Check sheet for the drawn part. Datum: minimum x, y, z corner. Units: mm. Coordinates: 2 decimals unless noted, no trailing zeros. Loops run counter-clockwise (first coordinate to the right, second up) from the corner with the lowest first, then second, coordinate; pieces in that order, holes last. Notation, with made-up numbers: M -12.5,33 L -6.5,33 A9 ccw -6.5,39 Z; hole C 64,5.25 d8. An arc over 180 degrees is marked long. Use CSV: the item, a comma, the result in double quotes. Start each with the question number.
(1) Section check B-B on x = 1.1. Record the cut outline in (y, z), and give its area (3 significant figures).
(2) Section check A-A on z = 0.5. Record the cut outline in (x, y), and give its area (3 significant figures).
(3) Scan lines: line 1 (Y direction, x = 0.75, z = 7.5); line 2 (X direction, y = 0.6, z = 3.5); line 3 (Y direction, x = 1.25, z = 7). Record each from-to range of solid material in increasing order.
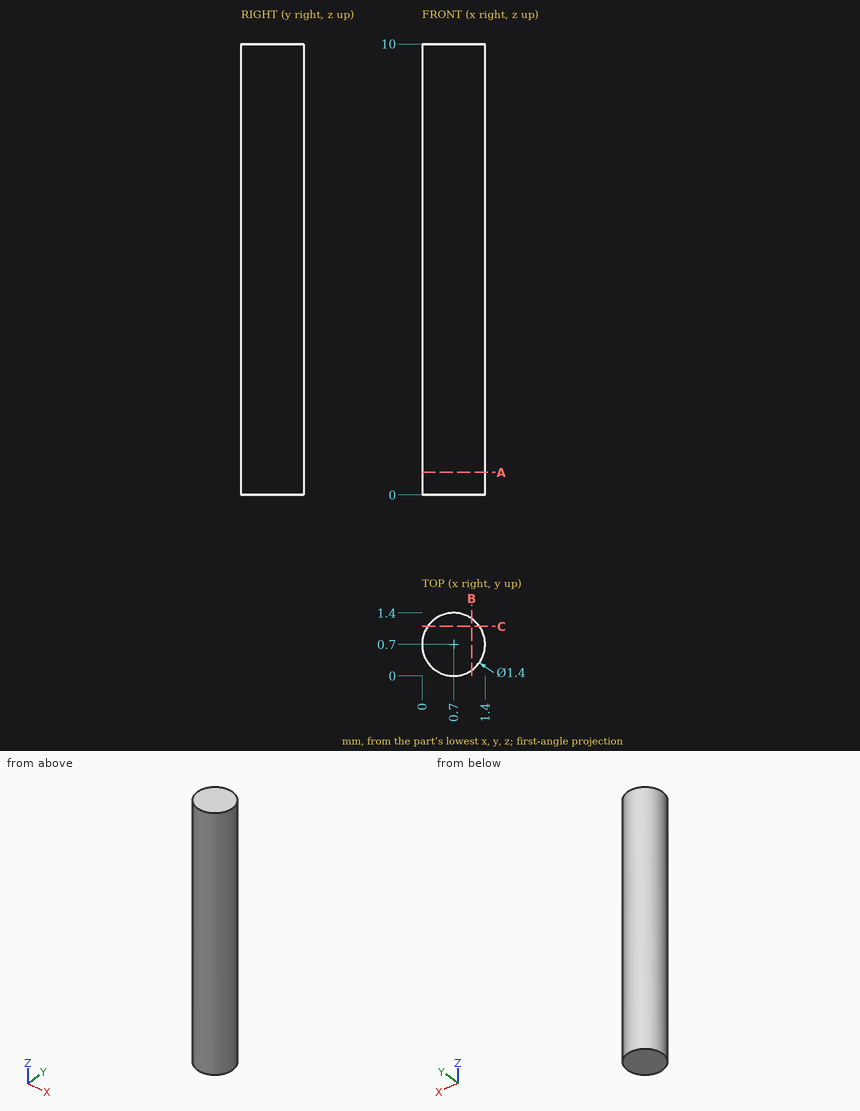
Outcome:
1,outline,"M 0.13,0 L 1.27,0 L 1.27,10 L 0.13,10 Z"
1,area,"11.5 mm²"
2,outline,"C 0.7,0.7 d1.4"
2,area,"1.54 mm²"
3,line 1,"y = 0 to 1.4"
3,line 2,"x = 0.01 to 1.39"
3,line 3,"y = 0.27 to 1.13"
